Input: part model. Units: mm. Frame: model coordinates. A direction names the side the tool comes from. Coordinates: 2 decimals unless noted, no trailing zeros. Loops run counter-clockwise (first coordinate to the right, second up) from the corner with the lowest first, then second, coordinate; pieces in that order, holes last. Notation, with made-up numbers: (85.25, 83.25) -> (97.25, 83.25) arc R18 cw to (97.25, 90.25) -> close; hole circle Ø2 at (49, 63.25). An arc over 180 degrees is marked (long way). Answer as a JSON object with one key per item and string values.
Autodesk Inventor part; units mm, degrees
ref_plane "YZ Plane" through (0, 0, 0) normal (1, 0, 0) x (0, 1, 0)
ref_plane "XZ Plane" through (0, 0, 0) normal (0, 1, 0) x (-1, 0, 0)
ref_plane "XY Plane" through (0, 0, 0) normal (0, 0, 1) x (1, 0, 0)
sketch "Sketch_1" plane through (0, 0, 0) normal (0, 0, 1) x (1, 0, 0)
  line L0 (30, 0) -> (0, 0)
  line L1 (0, 20) -> (0, 7.5)
  line L2 (0, 7.5) -> (30, 7.5)
  line L3 (30, 7.5) -> (30, 10)
  line L4 (30, 10) -> (6, 10)
  line L5 (6, 10) -> (6, 20)
  line L6 (6, 20) -> (0, 20)
revolve "Revolution1" add sketch "Sketch_1" angle 360 about axis through (30, 0, 0) along (1, 0, 0)
sketch "Sketch_3" plane through (0, 0, 0) normal (0, -0.7071, 0.7071) x (1, 0, 0)
  line L0 (18, 7) -> (18, 10)
  line L1 (18, 10) -> (20, 10)
  line L2 (20, 10) -> (19.621, 9.621)
  line L3 (19.621, 9.621) -> (19.621, 7)
  line L4 (19.621, 7) -> (18, 7)
  line L5 (18, 7) -> (18, 10)
revolve "Revolution2" cut sketch "Sketch_3" angle 360 about axis through (18, 4.9497, 4.9497) along (0, -0.7071, -0.7071)
thread "Thread1"
sketch "Sketch_2" plane through (0, 0, 0) normal (0, -0.7071, -0.7071) x (1, 0, 0)
  line L0 (18, 7) -> (18, 10)
  line L1 (18, 10) -> (20, 10)
  line L2 (20, 10) -> (19.621, 9.621)
  line L3 (19.621, 9.621) -> (19.621, 7)
  line L4 (19.621, 7) -> (18, 7)
  line L5 (18, 7) -> (18, 10)
revolve "Revolution3" cut sketch "Sketch_2" angle 360 about axis through (18, -4.9497, 4.9497) along (0, 0.7071, -0.7071)
thread "Thread2"
sketch "Sketch_4" plane through (0, 0, 0) normal (0, 0, 1) x (1, 0, 0)
  line L0 (6, 15) -> (0, 15)
  line L1 (0, 15) -> (0, 17)
  line L2 (0, 17) -> (0.379, 16.621)
  line L3 (0.379, 16.621) -> (5.621, 16.621)
  line L4 (5.621, 16.621) -> (6, 17)
  line L5 (6, 17) -> (6, 15)
  line L6 (6, 15) -> (0, 15)
revolve "Revolution4" cut sketch "Sketch_4" angle 360 about axis through (6, 15, 0) along (1, 0, 0)
thread "Thread3"
sketch "Sketch_9" plane through (0, 0, 0) normal (0, -1, 0) x (1, 0, 0)
  line L0 (0, -15) -> (6, -15)
  line L1 (6, -15) -> (6, -17)
  line L2 (6, -17) -> (5.621, -16.621)
  line L3 (5.621, -16.621) -> (0.379, -16.621)
  line L4 (0.379, -16.621) -> (0, -17)
  line L5 (0, -17) -> (0, -15)
  line L6 (0, -15) -> (6, -15)
revolve "Revolution5" cut sketch "Sketch_9" angle 360 about axis through (0, 0, -15) along (-1, 0, 0)
thread "Thread4"
sketch "Sketch_10" plane through (0, 0, 0) normal (0, 0, 1) x (1, 0, 0)
  line L0 (0, -15) -> (6, -15)
  line L1 (6, -15) -> (6, -17)
  line L2 (6, -17) -> (5.621, -16.621)
  line L3 (5.621, -16.621) -> (0.379, -16.621)
  line L4 (0.379, -16.621) -> (0, -17)
  line L5 (0, -17) -> (0, -15)
  line L6 (0, -15) -> (6, -15)
revolve "Revolution6" cut sketch "Sketch_10" angle 360 about axis through (0, -15, 0) along (-1, 0, 0)
thread "Thread5"
sketch "Sketch_11" plane through (0, 0, 0) normal (0, -1, 0) x (1, 0, 0)
  line L0 (6, 15) -> (0, 15)
  line L1 (0, 15) -> (0, 17)
  line L2 (0, 17) -> (0.379, 16.621)
  line L3 (0.379, 16.621) -> (5.621, 16.621)
  line L4 (5.621, 16.621) -> (6, 17)
  line L5 (6, 17) -> (6, 15)
  line L6 (6, 15) -> (0, 15)
revolve "Revolution7" cut sketch "Sketch_11" angle 360 about axis through (6, 0, 15) along (1, 0, 0)
thread "Thread6"
properties part number "STHRBT15_b" material "ステンレス鋼"
1. Pin query (flat end, axial travel): P1, Ø8, axis at x = 13.5, y = -2.5, coming from the -Z side; P2, Ø2, axis at x = 11.5, z = -0.5, coming from the -Y side; P3, Ø1.9, axis at y = 15, z = 0, coming from the +X side; P4, Ø1, axis at y = 15, z = -10, coming from the +X side. Return the tip coordinate at first contact, or that it passes through.
Reply:
{"P1": "stops at z = -10", "P2": "stops at y = -10", "P3": "passes through", "P4": "stops at x = 6"}
2. Access query for faces 4 (the face through (17.83, 9.54, -3)), 5 (the face through (15.21, 6.93, -2.87)). Directions: +Z, -Z, +X, -X, +Y, -Y. A direction counts if a zero-diameter tool reaches every point of the face in a straight line with its end or side. Return the directions, or none.
Reply:
{"face 4": "+X", "face 5": "+X, -X"}
3. Section query A-A (y = 0). Return loops of the section in (x, z), plus the area to 3 significant figures.
Reply:
{"outline": "(0, -20) -> (6, -20) -> (6, -17) -> (5.62, -16.62) -> (0.38, -16.62) -> (0, -17) -> close; (0, -13) -> (0.38, -13.38) -> (5.62, -13.38) -> (6, -13) -> (6, -10) -> (30, -10) -> (30, -7.5) -> (0, -7.5) -> close; (0, 7.5) -> (30, 7.5) -> (30, 10) -> (6, 10) -> (6, 13) -> (5.62, 13.38) -> (0.38, 13.38) -> (0, 13) -> close; (0, 17) -> (0.38, 16.62) -> (5.62, 16.62) -> (6, 17) -> (6, 20) -> (0, 20) -> close", "area": "231 mm2"}
4. Section query B-B (z = -3). Return loops of the section in (x, y).
Reply:
{"outline": "(0, -19.77) -> (6, -19.77) -> (6, -9.54) -> (30, -9.54) -> (30, -6.87) -> (0, -6.87) -> close; (0, 6.87) -> (30, 6.87) -> (30, 9.54) -> (6, 9.54) -> (6, 19.77) -> (0, 19.77) -> close"}
5. Mould query, pull axis Z, two halves, no side actions, for faces 1 (the face through (2.958, -4.336, 19.524)), 2 (the face through (2.963, -16.546, 0.487)), 3 (the face through (6, -5, 9)). Classes: pulls with the +Z half, pulls with the -Z half, needs draft (parallel to the pull), parting line crosses it, or undercut.
Reply:
{"face 1": "parting line crosses it", "face 2": "undercut", "face 3": "needs draft"}
6. Section query C-C (x = 3.5). Return loops of the section in (y, z).
Reply:
{"outline": "circle Ø40 at (0, 0); hole circle Ø3.24 at (-15, 0); hole circle Ø15 at (0, 0); hole circle Ø3.24 at (0, -15); hole circle Ø3.24 at (0, 15); hole circle Ø3.24 at (15, 0)"}
7. Line query: line 1 along Z through (x, y) = (3.65, 0); line 2 along Z through (x, y) = (14.5, 0); line 3 along X through (y, z) = (16, -4). Output: solid intervals per line, ascending.
Reply:
{"line 1": "z = -20 to -16.62, -13.38 to -7.5, 7.5 to 13.38, 16.62 to 20", "line 2": "z = -10 to -7.5, 7.5 to 10", "line 3": "x = 0 to 6"}
8. Section query D-D (y = 15). Return loops of the section in (x, z).
Reply:
{"outline": "(0, -13.23) -> (6, -13.23) -> (6, -2) -> (5.62, -1.62) -> (0.38, -1.62) -> (0, -2) -> close; (0, 2) -> (0.38, 1.62) -> (5.62, 1.62) -> (6, 2) -> (6, 13.23) -> (0, 13.23) -> close"}
